Model file for the job. Use its own axes, mm. Coordinates: 2 decimals unless noted, no trailing zeros. Order: outer loops, then holes, each group sorted by start corner. A loop starts at its lowest first (then second) coordinate and runs counter-clockwise, first axis right, second up. Notation, with made-up numbers: M 53,-32 L 64,-32 A18 ccw 64,-18 Z; hole C 26,-25 d10. An arc over 180 degrees is marked long. Return JSON: item names as keys, results as strings.
```python
from build123d import *

# Parameters (mm, degrees)
SKETCH1_W           = 193
SKETCH1_H           = 124
SKETCH1_R           = 1.5
BOSS_EXTRUDE1_DEPTH = 3
SKETCH2_R           = 3
SKETCH2_R_2         = 2.5
SKETCH2_R_3         = 6
SKETCH2_W           = 35
SKETCH2_H           = 7
SKETCH2_W_2         = 21
SKETCH2_H_2         = 16
SKETCH2_W_3         = 6
SKETCH2_H_3         = 21
SKETCH2_W_4         = 8
SKETCH2_H_4         = 12
CUT_EXTRUDE1_DEPTH  = 230.421010372
SKETCH3_R           = 11
SKETCH3_R_2         = 6.5
CUT_EXTRUDE2_DEPTH  = 230.421010372
SKETCH4_W           = 10
SKETCH4_H           = 6
CUT_EXTRUDE3_DEPTH  = 230.421010372
SKETCH5_W           = 30
SKETCH5_H           = 4
CUT_EXTRUDE4_DEPTH  = 230.421010372
SKETCH6_R           = 1.5
SKETCH6_W           = 4
SKETCH6_H           = 18
CUT_EXTRUDE5_DEPTH  = 230.421010372
SKETCH7_W           = 6
SKETCH7_H           = 10
CUT_EXTRUDE6_DEPTH  = 230.421010372
FILLET1_R           = 2


with BuildPart() as part:
    # Sketch1 → Boss-Extrude1 (new body)
    with BuildSketch(Plane(origin=(0, 0, 0), x_dir=(1, 0, 0), z_dir=(0, 1, 0))):
        with Locations((96.5, 62)):
            Rectangle(SKETCH1_W, SKETCH1_H)
        with Locations(Location((13, 119, 0), (0, 0, 270))):
            Circle(SKETCH1_R, mode=Mode.SUBTRACT)
        with Locations(Location((178, 119, 0), (0, 0, 270))):
            Circle(SKETCH1_R, mode=Mode.SUBTRACT)
        with Locations(Location((13, 5, 0), (0, 0, 270))):
            Circle(SKETCH1_R, mode=Mode.SUBTRACT)
        with Locations(Location((178, 5, 0), (0, 0, 270))):
            Circle(SKETCH1_R, mode=Mode.SUBTRACT)
    extrude(amount=BOSS_EXTRUDE1_DEPTH)

    # Sketch2 → Cut-Extrude1 (cut, through all)
    with BuildSketch(Plane(origin=(0, 3, 0), x_dir=(1, 0, 0), z_dir=(0, 1, 0))):
        with Locations(Location((157, 80, 0), (0, 0, 270))):
            Circle(SKETCH2_R)
        with Locations(Location((161, 74.255437353, 0), (0, 0, 270))):
            Circle(SKETCH2_R)
        with Locations(Location((159, 64, 0), (0, 0, 270))):
            Circle(SKETCH2_R)
        with Locations(Location((181, 85, 0), (0, 0, 270))):
            Circle(SKETCH2_R_2)
        with Locations(Location((176, 24, 0), (0, 0, 270))):
            Circle(SKETCH2_R_3)
        with Locations((153.5, 39.5)):
            Rectangle(SKETCH2_W, SKETCH2_H)
        with Locations((137, 86.5)):
            Rectangle(SKETCH2_W_2, SKETCH2_H_2)
        with Locations((176, 72.5)):
            Rectangle(SKETCH2_W_3, SKETCH2_H_3)
        with Locations((127, 37)):
            Rectangle(SKETCH2_W_4, SKETCH2_H_4)
    extrude(amount=-CUT_EXTRUDE1_DEPTH, mode=Mode.SUBTRACT)

    # Sketch3 → Cut-Extrude2 (cut, through all)
    with BuildSketch(Plane(origin=(0, 3, 0), x_dir=(1, 0, 0), z_dir=(0, 1, 0))):
        with Locations(Location((93, 77, 0), (0, 0, 270))):
            Circle(SKETCH3_R)
        with Locations(Location((93, 47, 0), (0, 0, 270))):
            Circle(SKETCH3_R_2)
    extrude(amount=-CUT_EXTRUDE2_DEPTH, mode=Mode.SUBTRACT)

    # Sketch4 → Cut-Extrude3 (cut, through all)
    with BuildSketch(Plane(origin=(0, 3, 0), x_dir=(1, 0, 0), z_dir=(0, 1, 0))):
        with Locations((29, 113)):
            Rectangle(SKETCH4_W, SKETCH4_H)
        with Locations((159, 113)):
            Rectangle(SKETCH4_W, SKETCH4_H)
        with Locations((29, 11)):
            Rectangle(SKETCH4_W, SKETCH4_H)
        with Locations((159, 11)):
            Rectangle(SKETCH4_W, SKETCH4_H)
    extrude(amount=-CUT_EXTRUDE3_DEPTH, mode=Mode.SUBTRACT)

    # Sketch5 → Cut-Extrude4 (cut, through all)
    with BuildSketch(Plane(origin=(0, 3, 0), x_dir=(1, 0, 0), z_dir=(0, 1, 0))):
        with Locations((65, 2)):
            Rectangle(SKETCH5_W, SKETCH5_H)
    extrude(amount=-CUT_EXTRUDE4_DEPTH, mode=Mode.SUBTRACT)

    # Sketch6 → Cut-Extrude5 (cut, through all)
    with BuildSketch(Plane(origin=(0, 3, 0), x_dir=(1, 0, 0), z_dir=(0, 1, 0))):
        with Locations(Location((8.5, 56, 0), (0, 0, 270))):
            Circle(SKETCH6_R)
        with Locations(Location((22.5, 68, 0), (0, 0, 270))):
            Circle(SKETCH6_R)
        with Locations((27, 62)):
            Rectangle(SKETCH6_W, SKETCH6_H)
    extrude(amount=-CUT_EXTRUDE5_DEPTH, mode=Mode.SUBTRACT)

    # Sketch7 → Cut-Extrude6 (cut, through all)
    with BuildSketch(Plane(origin=(0, 3, 0), x_dir=(1, 0, 0), z_dir=(0, 1, 0))):
        with Locations((13, 35)):
            Rectangle(SKETCH7_W, SKETCH7_H)
        with Locations((49, 35)):
            Rectangle(SKETCH7_W, SKETCH7_H)
    extrude(amount=-CUT_EXTRUDE6_DEPTH, mode=Mode.SUBTRACT)

    # Fillet1
    fillet1_edges = [part.edges().sort_by_distance(p)[0] for p in [
        (0, 1.5, -124),
        (193, 1.5, -124),
        (193, 1.5, 0),
        (0, 1.5, 0),
    ]]
    fillet(fillet1_edges, radius=FILLET1_R)


solid = part.part
```
Item 1: Drop a flat-ended pin along its axis: pin 1 Ø1 at (x, y) = (75.5, 2.5) entering from +Z. Give the stop position or say it passes through.
Check result:
{"pin 1": "stops at z = -4"}
Item 2: Pull direction X, two halves, no side cores. Call faces 1 (the flat face through (95, 0, -63)), 2 (the cylindrical face through (183.48, 1.52, -85.33)): +X half, -X half, draft (parallel to the pull), parting line (faces both ways), or undercut.
Check result:
{"face 1": "draft", "face 2": "undercut"}
Item 3: Saw through at C-C (z = -47). Write the cut outline in (x, y), and give its area (3 significant figures).
Check result:
{"outline": "M 0,0 L 86.5,0 L 86.5,3 L 0,3 Z; M 99.5,0 L 193,0 L 193,3 L 99.5,3 Z", "area": "540 mm2"}
Item 4: Wall check: line 1 (X direction, y = 1.5, z = -34); line 2 (Z direction, x = 141.5, y = 0.1); line 3 (X direction, y = 1.8, z = -113). Give the ranges that are in metal, low to high.
Check result:
{"line 1": "x = 0 to 10, 16 to 46, 52 to 123, 131 to 193", "line 2": "z = -124 to -94.5, -78.5 to -43, -36 to 0", "line 3": "x = 0 to 24, 34 to 154, 164 to 193"}
Item 5: Saw through at D-D (z = -11.5). Write the cut outline in (x, y), and give its area (3 significant figures).
Check result:
{"outline": "M 0,0 L 24,0 L 24,3 L 0,3 Z; M 34,0 L 154,0 L 154,3 L 34,3 Z; M 164,0 L 193,0 L 193,3 L 164,3 Z", "area": "519 mm2"}
Item 6: Saw through at A-A (z = -64). Write the cut outline in (x, y).
Check result:
{"outline": "M 0,0 L 25,0 L 25,3 L 0,3 Z; M 29,0 L 156,0 L 156,3 L 29,3 Z; M 162,0 L 173,0 L 173,3 L 162,3 Z; M 179,0 L 193,0 L 193,3 L 179,3 Z"}
Item 7: Saw through at B-B (x = 93). Write the cut outline in (y, z).
Check result:
{"outline": "M 0,-124 L 3,-124 L 3,-88 L 0,-88 Z; M 0,-66 L 3,-66 L 3,-53.5 L 0,-53.5 Z; M 0,-40.5 L 3,-40.5 L 3,0 L 0,0 Z"}
